CAD build for the part. Positions are in the model's coordinates, mm. Round coordinates to 2 decimals unless told otherwise and drop trailing zeros. Loops run counter-clockwise (first coordinate to the right, second up) from the corner with the lowest first, then second, coordinate; pieces in that order, holes last. Notation, with made-up numbers: (79, 53) - (116, 53) arc R28 cw to (116, 83) - close; hole circle Ø6 at (27.5, -0.5). An arc over 180 degrees is marked (long way). One line per question, with ' | ' between items.
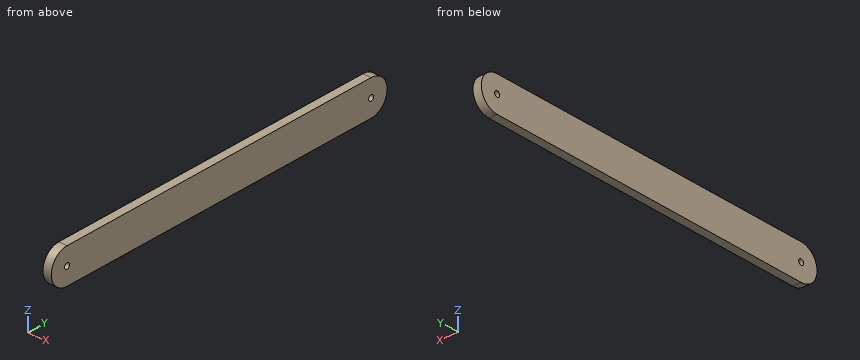
Autodesk Inventor part; units mm, degrees
ref_plane "YZ Plane" through (0, 0, 0) normal (1, 0, 0) x (0, 1, 0)
ref_plane "XZ Plane" through (0, 0, 0) normal (0, 1, 0) x (-1, 0, 0)
ref_plane "XY Plane" through (0, 0, 0) normal (0, 0, 1) x (1, 0, 0)
sketch "Sketch1" plane through (0, 0, 0) normal (0, 0, 1) x (1, 0, 0)
  line L0 (0, 0) -> (-25, 0)
  line L1 (-25, 0) -> (-25, 265)
  line L2 (-25, 265) -> (0, 265)
  line L3 (0, 265) -> (0, 0)
  dimension "d0" = 265
  dimension "d1" = 25
extrude "Extrusion1" add sketch "Sketch1" along normal blind 25
sketch "Sketch2" plane through (0, 0, 0) normal (1, 0, 0) x (0, 0, -1)
  circle A0 centre (-12.5, 12.5) radius 12.5
  line L0 (0, 0) -> (-25, 0)
  circle A1 centre (-12.5, 12.5) radius 2
  circle A2 centre (-12.5, 252.5) radius 12.5
  line L1 (0, 265) -> (-25, 265)
  circle A3 centre (-12.5, 252.5) radius 2
  line L2 (0, 0) -> (0, 265)
  line L3 (-25, 0) -> (-25, 265)
  point P0 (-12.5, 0)
  point P1 (-25, 252.5)
  point P2 (-12.5, 265)
  point P3 (0, 252.5)
  point P4 (-25, 12.5)
  point P5 (-12.5, 0)
  point P6 (0, 12.5)
  dimension "d4" = 25
  dimension "d5" = 12.5
  dimension "d6" = 4
  dimension "d7" = 25
  dimension "d8" = 12.5
  dimension "d9" = 4
  dimension "d10" = 12.5
  dimension "d11" = 12.5
extrude "Extrusion2" cut sketch "Sketch2" against normal blind 25 contours L2 L0 A0 | A0 L0 L3 | A2 L1 L2 | L3 L1 A2 | A1 | A3
sketch "Sketch3" plane through (0, 0, 25) normal (0, 0, 1) x (1, 0, 0)
  line L0 (-25, 265) -> (0, 265)
  line L1 (0, 0) -> (-19, 0)
  line L2 (-19, 0) -> (-19, 265)
  line L3 (-19, 265) -> (0, 265)
  line L4 (0, 265) -> (0, 0)
  point P0 (0, 265)
  dimension "d14" = 19
extrude "Extrusion3" cut sketch "Sketch3" against normal blind 100
properties part number "Vertical"
(1) Drop a flat-ended pin along its axis: P1, Ø3, axis at x = -20, z = 15.5, coming from the -Y side. Give the stop position or say it passes through.
Results found:
P1: stops at y = 0.09
(2) Cut at C-C, the plane z = 3.25. Write the cut outline in (x, y).
Results found:
outline: (-25, 4.09) - (-19, 4.09) - (-19, 260.91) - (-25, 260.91) - close
(3) Cut at A-A, the plane x = -20.25. Write the cut outline in (y, z).
Results found:
outline: (12.5, 0) - (252.5, 0) arc R12.5 ccw to (252.5, 25) - (12.5, 25) arc R12.5 ccw to start; hole circle Ø4 at (12.5, 12.5); hole circle Ø4 at (252.5, 12.5)
(4) Cut at B-B, the plane z = 21.25. Write the cut outline in (x, y), then the cut area to 3 significant figures.
Results found:
outline: (-25, 3.57) - (-19, 3.57) - (-19, 261.43) - (-25, 261.43) - close | area: 1,550 mm²
(5) Probe L1, parallel to Y at x = -22.85, z = 12.5; L2, parallel to Z at x = -21, y = 252.5; L3, parallel to Y at x = -23.6, z = 2.25. List the from-to ranges inside material, lowest first.
Results found:
L1: y = 0 to 10.5, 14.5 to 250.5, 254.5 to 265 | L2: z = 0 to 10.5, 14.5 to 25 | L3: y = 5.35 to 259.65
